For this review, take the finished solid that the model builds, in its own axes (mm). Coordinates: 2 decimals unless noted, no trailing zeros. Write each loop counter-clockwise with the first axis right and the second up, starting at its lowest first coordinate (ties: lowest second). Pieces come first, ordered by that corner, then holes. Notation, with made-up numbers: (31.5, -0.5) -> (74.5, -0.5) arc R27 cw to (74.5, 21.5) -> close; hole circle Ø9 at (50, -27.5). An arc over 180 degrees is marked (long way). Put each result on its own line as item: value. Start each with the question number.
Item 1: Consider section A-A on y = -1.2. Give the number of separate pieces and of enclosed holes in the cut face, and give its area (3 significant figures).
Item 2: Consider section B-B on z = -31.5. Give the boundary of the cut face in (x, y) (3 decimals).
Item 3: Insertion check: P1, Ø4, axis at x = 36.53, z = 3.18, coming from the -Y side; P2, Ø1, axis at y = -1, z = 6.5, coming from the -X side; P3, Ø1.5, axis at x = 21, y = -1, coming from the +Z side; P4, Ø1.5, axis at x = -44, y = -1, coming from the +Z side. Each pin has a flat end and moves straight along its axis. Give the tip position at first contact, or say it passes through.
Item 4: To check wall thickness, follow L1, parallel to X at y = -0.75, z = -45.5; L2, parallel to X at y = -1.6, z = -42; L3, parallel to Z at x = 50.8, y = -2.5 (3 decimals). State the ranges of each line that lie inside material, in increasing order.
```python
from build123d import *

# Parameters (mm, degrees)
F1_DEPTH = 3.175


with BuildPart() as f1:
    # F0 (on Front) → F1 (new body)
    with BuildSketch(Plane.XZ):
        with BuildLine():
            Line((15.875, 0), (3.9751, 0))
            ThreePointArc((3.9751, 0), (0, -3.9751), (-3.9751, 0))
            Line((-3.9751, 0), (-15.875, 0))
            ThreePointArc((-15.875, 0), (-10.6817358486, -11.7437704448), (1.5002622689, -15.8039500798))
            ThreePointArc((1.5002622689, -15.8039500798), (11.7437704448, -10.6817358486), (15.875, 0))
        make_face()
        with BuildLine():
            ThreePointArc((-3.9751, 0), (0, 3.9751), (3.9751, 0))
            Line((3.9751, 0), (15.875, 0))
            ThreePointArc((15.875, 0), (12.0288225692, 10.3596840009), (2.3539854993, 15.6995024529))
            Line((2.3539854993, 15.6995024529), (0.6027935511, 15.8635514603))
            ThreePointArc((0.6027935511, 15.8635514603), (-0.2955948224, 15.872247752), (-1.1930364393, 15.8301070449))
            ThreePointArc((-1.1930364393, 15.8301070449), (-11.6394819145, 10.7952807172), (-15.875, 0))
            Line((-15.875, 0), (-3.9751, 0))
        make_face()
        with BuildLine():
            Line((36.5252, 0), (15.875, 0))
            ThreePointArc((15.875, 0), (11.7437704448, -10.6817358486), (1.5002622689, -15.8039500798))
            Line((1.5002622689, -15.8039500798), (50.9283921277, -11.1117582637))
            ThreePointArc((50.9283921277, -11.1117582637), (42.9878012464, -7.9029872127), (39.6875, 0))
            Line((39.6875, 0), (36.5252, 0))
        make_face()
        with BuildLine():
            ThreePointArc((2.3539854993, 15.6995024529), (12.0288225692, 10.3596840009), (15.875, 0))
            Line((15.875, 0), (36.5252, 0))
            Line((36.5252, 0), (39.6875, 0))
            ThreePointArc((39.6875, 0), (43.3176892897, 8.2160016239), (51.8364642626, 11.064058843))
            Line((51.8364642626, 11.064058843), (2.3539854993, 15.6995024529))
        make_face()
        with BuildLine():
            ThreePointArc((39.7002, 3.175), (38.7702640303, 0.9299359697), (36.5252, 0))
            ThreePointArc((36.5252, 0), (34.2801359697, 5.4200640303), (39.7002, 3.175))
        make_face(mode=Mode.SUBTRACT)
        with BuildLine():
            Line((-52.3875, 0), (-15.875, 0))
            ThreePointArc((-15.875, 0), (-11.6394819145, 10.7952807172), (-1.1930364393, 15.8301070449))
            Line((-1.1930364393, 15.8301070449), (-63.8728285154, 11.1062439712))
            ThreePointArc((-63.8728285154, 11.1062439712), (-55.7752152337, 7.9884514497), (-52.3875, 0))
        make_face()
        with BuildLine():
            ThreePointArc((1.5002622689, -15.8039500798), (-10.6817358486, -11.7437704448), (-15.875, 0))
            Line((-15.875, 0), (-52.3875, 0))
            ThreePointArc((-52.3875, 0), (-52.4153874044, -0.7867781489), (-52.4989096478, -1.5696073753))
            ThreePointArc((-52.4989096478, -1.5696073753), (-56.2183314312, -8.3943408975), (-63.5, -11.1125))
            Line((-63.5, -11.1125), (-63.5, -36.5125))
            ThreePointArc((-63.5, -36.5125), (-57.8873399243, -38.8373399243), (-55.5625, -44.45))
            ThreePointArc((-55.5625, -44.45), (-55.5674814568, -44.7311686533), (-55.5824195746, -45.0119843921))
            Line((-55.5824195746, -45.0119843921), (-53.7975104819, -19.8650915378))
            ThreePointArc((-53.7975104819, -19.8650915378), (-51.0613936601, -14.4091151142), (-45.2638074239, -12.5007105892))
            Line((-45.2638074239, -12.5007105892), (0, -15.9463693532))
            Line((0, -15.9463693532), (1.5002622689, -15.8039500798))
        make_face()
        with BuildLine():
            Line((0.6027935511, 15.8635514603), (2.3539854993, 15.6995024529))
            ThreePointArc((2.3539854993, 15.6995024529), (1.4806632323, 15.8057983472), (0.6027935511, 15.8635514603))
        make_face()
        with BuildLine():
            Line((0, 15.9200202465), (-1.1930364393, 15.8301070449))
            ThreePointArc((-1.1930364393, 15.8301070449), (-0.2955948224, 15.872247752), (0.6027935511, 15.8635514603))
            Line((0.6027935511, 15.8635514603), (0, 15.9200202465))
        make_face()
        with BuildLine():
            Line((-60.325, 0), (-52.3875, 0))
            ThreePointArc((-52.3875, 0), (-55.7752152337, 7.9884514497), (-63.8728285154, 11.1062439712))
            ThreePointArc((-63.8728285154, 11.1062439712), (-71.4884514497, 7.7247847663), (-74.6125, 0))
            Line((-74.6125, 0), (-74.5010903522, -1.5696073753))
            ThreePointArc((-74.5010903522, -1.5696073753), (-70.7816685688, -8.3943408975), (-63.5, -11.1125))
            Line((-63.5, -11.1125), (-63.5, -3.175))
            ThreePointArc((-63.5, -3.175), (-65.7450640303, 2.2450640303), (-60.325, 0))
        make_face()
        with BuildLine():
            ThreePointArc((61.9125, 0), (59.0160016239, 7.4823107103), (51.8364642626, 11.064058843))
            ThreePointArc((51.8364642626, 11.064058843), (43.3176892897, 8.2160016239), (39.6875, 0))
            ThreePointArc((39.6875, 0), (42.9878012464, -7.9029872127), (50.9283921277, -11.1117582637))
            ThreePointArc((50.9283921277, -11.1117582637), (58.7029872127, -7.8121987536), (61.9125, 0))
        make_face()
        with BuildLine():
            ThreePointArc((53.975, 0), (50.8, -3.175), (47.625, 0))
            ThreePointArc((47.625, 0), (50.8, 3.175), (53.975, 0))
        make_face(mode=Mode.SUBTRACT)
        with BuildLine():
            Line((-74.5010903522, -1.5696073753), (-74.6125, 0))
            ThreePointArc((-74.6125, 0), (-74.5846125956, -0.7867781489), (-74.5010903522, -1.5696073753))
        make_face()
        with BuildLine():
            Line((-63.5, -36.5125), (-63.5, -11.1125))
            ThreePointArc((-63.5, -11.1125), (-70.7816685688, -8.3943408975), (-74.5010903522, -1.5696073753))
            Line((-74.5010903522, -1.5696073753), (-71.4175804254, -45.0119843921))
            ThreePointArc((-71.4175804254, -45.0119843921), (-69.3079539152, -39.0396786076), (-63.5, -36.5125))
        make_face()
        with BuildLine():
            ThreePointArc((-55.5625, -44.45), (-57.8873399243, -38.8373399243), (-63.5, -36.5125))
            ThreePointArc((-63.5, -36.5125), (-69.3079539152, -39.0396786076), (-71.4175804254, -45.0119843921))
            ThreePointArc((-71.4175804254, -45.0119843921), (-63.5, -52.3875), (-55.5824195746, -45.0119843921))
            ThreePointArc((-55.5824195746, -45.0119843921), (-55.5674814568, -44.7311686533), (-55.5625, -44.45))
        make_face()
        with BuildLine():
            ThreePointArc((-60.325, -44.45), (-65.7450640303, -46.6950640303), (-63.5, -41.275))
            ThreePointArc((-63.5, -41.275), (-61.2549359697, -42.2049359697), (-60.325, -44.45))
        make_face(mode=Mode.SUBTRACT)
        with BuildLine():
            Line((-52.4989096478, -1.5696073753), (-52.3875, 0))
            Line((-52.3875, 0), (-60.325, 0))
            ThreePointArc((-60.325, 0), (-61.2549359697, -2.2450640303), (-63.5, -3.175))
            Line((-63.5, -3.175), (-63.5, -11.1125))
            ThreePointArc((-63.5, -11.1125), (-56.2183314312, -8.3943408975), (-52.4989096478, -1.5696073753))
        make_face()
    extrude(amount=F1_DEPTH)


solid = f1.part
```
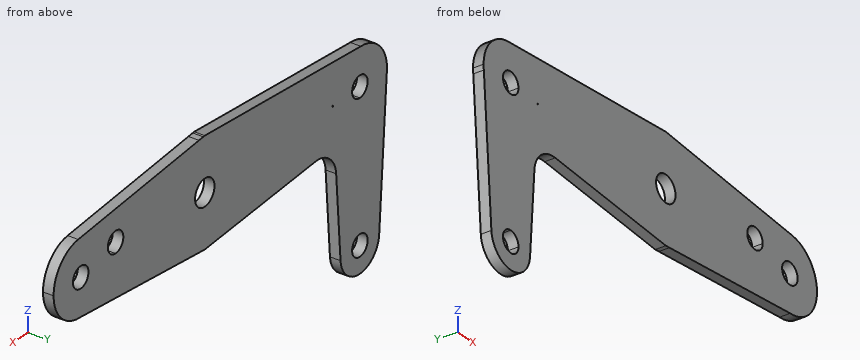
Return value:
1. separate pieces: 1
1. enclosed holes: 6
1. area: 4,050 mm^2
2. outline: (-72.377, -3.175) -> (-54.623, -3.175) -> (-54.623, 0) -> (-72.377, 0) -> close
3. P1: through
3. P2: x = -72.85
3. P3: z = 14.02
3. P4: z = 12.66
4. L1: -71.37 to -66.5, -60.5 to -55.63
4. L2: -71.63 to -65.52, -61.48 to -55.37
4. L3: -11.124 to -3.175, 3.175 to 11.161
